```python
from build123d import *

# Parameters (mm, degrees)
SKETCH_1_R               = 275
SKETCH_1_R_2             = 255
EXTRUDE_1_DEPTH          = 10
EXTRUDE_2_DEPTH          = 10
SKETCH_8_R               = 2.65
SKETCH_8_R_2             = 2.15
CUT_EXTRUDE_1_DEPTH      = 21
SKETCH_9_OUTSIDE_W       = 707.614
SKETCH_9_OUTSIDE_H       = 707.614
CUT_EXTRUDE_2_DEPTH      = 21
SKETCH_10_W              = 190.987823936
SKETCH_10_H              = 12
CUT_EXTRUDE_3_DEPTH      = 519.420037555
CUT_EXTRUDE_3_DEPTH_BACK = 245.939436413
FILLET_1_R               = 3
FILLET_2_R               = 10
FILLET_3_R               = 5
SKETCH_11_W              = 751.740061758
SKETCH_11_H              = 25.075171634
CUT_EXTRUDE_4_DEPTH      = 519.420037555
CUT_EXTRUDE_4_DEPTH_BACK = 245.939436413


with BuildPart() as part:
    # 草图1 → 凸台-拉伸1 (new body)
    with BuildSketch(Plane(origin=(0, 0, 0), x_dir=(1, 0, 0), z_dir=(0, 1, 0))):
        Circle(SKETCH_1_R)
        Circle(SKETCH_1_R_2, mode=Mode.SUBTRACT)
    extrude(amount=EXTRUDE_1_DEPTH)

    # 草图11 → 切除-拉伸4 (cut, two sides)
    with BuildSketch(Plane(origin=(76.33674701, 0, -113.448714652), x_dir=(0.829665535, 0, 0.558260781), z_dir=(-0.558260781, 0, 0.829665535))) as cut_extrude_4_sk:
        with Locations((71.776229786, 3.462414183)):
            Rectangle(SKETCH_11_W, SKETCH_11_H)
    extrude(amount=CUT_EXTRUDE_4_DEPTH, mode=Mode.SUBTRACT)
    extrude(cut_extrude_4_sk.sketch, amount=-CUT_EXTRUDE_4_DEPTH_BACK, mode=Mode.SUBTRACT)


with BuildPart() as body_2:
    # 草图2 → 凸台-拉伸2 (new body)
    with BuildSketch(Plane(origin=(0, 10, 0), x_dir=(1, 0, 0), z_dir=(0, 1, 0))):
        with BuildLine():
            Line((-110.525139894, 257.262887824), (-25.423255477, 200))
            Line((-25.423255477, 200), (0, 200))
            Line((0, 200), (25.423255477, 200))
            Line((25.423255477, 200), (110.525139894, 257.262887824))
            ThreePointArc((110.525139894, 257.262887824), (197.989898732, 197.989898732), (257.262887824, 110.525139894))
            Line((257.262887824, 110.525139894), (200, 25.423255477))
            Line((200, 25.423255477), (200, 0))
            Line((200, 0), (200, -25.423255477))
            Line((200, -25.423255477), (257.262887824, -110.525139894))
            ThreePointArc((257.262887824, -110.525139894), (197.989898732, -197.989898732), (110.525139894, -257.262887824))
            Line((110.525139894, -257.262887824), (25.423255477, -200))
            Line((25.423255477, -200), (0, -200))
            Line((0, -200), (-25.423255477, -200))
            Line((-25.423255477, -200), (-110.525139894, -257.262887824))
            ThreePointArc((-110.525139894, -257.262887824), (-197.989898732, -197.989898732), (-257.262887824, -110.525139894))
            Line((-257.262887824, -110.525139894), (-200, -25.423255477))
            Line((-200, -25.423255477), (-200, 25.423255477))
            Line((-200, 25.423255477), (-257.262887824, 110.525139894))
            ThreePointArc((-257.262887824, 110.525139894), (-197.989898732, 197.989898732), (-110.525139894, 257.262887824))
        make_face()
        with BuildLine():
            Line((0, 185), (30, 185))
            Line((30, 185), (111.993839361, 240.171563565))
            ThreePointArc((111.993839361, 240.171563565), (187.383297014, 187.383297014), (240.171563565, 111.993839361))
            Line((240.171563565, 111.993839361), (185, 30))
            Line((185, 30), (185, 0))
            Line((185, 0), (185, -30))
            Line((185, -30), (240.171563565, -111.993839361))
            ThreePointArc((240.171563565, -111.993839361), (187.383297014, -187.383297014), (111.993839361, -240.171563565))
            Line((111.993839361, -240.171563565), (30, -185))
            Line((30, -185), (0, -185))
            Line((0, -185), (-30, -185))
            Line((-30, -185), (-111.993839361, -240.171563565))
            ThreePointArc((-111.993839361, -240.171563565), (-187.383297014, -187.383297014), (-240.171563565, -111.993839361))
            Line((-240.171563565, -111.993839361), (-185, -30))
            Line((-185, -30), (-185, 30))
            Line((-185, 30), (-240.171563565, 111.993839361))
            ThreePointArc((-240.171563565, 111.993839361), (-187.383297014, 187.383297014), (-111.993839361, 240.171563565))
            Line((-111.993839361, 240.171563565), (-30, 185))
            Line((-30, 185), (0, 185))
        make_face(mode=Mode.SUBTRACT)
    extrude(amount=EXTRUDE_2_DEPTH)

    # 草图8 → 切除-拉伸1 (cut, through all)
    with BuildSketch(Plane(origin=(0, 20, 0), x_dir=(1, 0, 0), z_dir=(0, 1, 0))):
        with Locations((-10, 192.5)):
            Circle(SKETCH_8_R)
        with Locations((10, 192.5)):
            Circle(SKETCH_8_R)
        with Locations((-10, -192.5)):
            Circle(SKETCH_8_R)
        with Locations((10, -192.5)):
            Circle(SKETCH_8_R)
        with Locations((192.5, 10)):
            Circle(SKETCH_8_R)
        with Locations((192.5, -10)):
            Circle(SKETCH_8_R)
        with Locations((-192.5, 10)):
            Circle(SKETCH_8_R)
        with Locations((-192.5, -10)):
            Circle(SKETCH_8_R)
        with Locations((-110.525139894, 248.223100485)):
            Circle(SKETCH_8_R_2)
        with Locations((-27.711627738, 192.5)):
            Circle(SKETCH_8_R_2)
        with Locations((-44.304938442, 203.665215623)):
            Circle(SKETCH_8_R_2)
        with Locations((-56.749921469, 212.03912734)):
            Circle(SKETCH_8_R_2)
        with Locations((-69.194904497, 220.413039057)):
            Circle(SKETCH_8_R_2)
        with Locations((-81.639887524, 228.786950774)):
            Circle(SKETCH_8_R_2)
        with Locations((-146.077022117, 230.028561882)):
            Circle(SKETCH_8_R_2)
        with Locations((-164.415519771, 217.299729706)):
            Circle(SKETCH_8_R_2)
        with Locations((-183.638937552, 201.316607082)):
            Circle(SKETCH_8_R_2)
        with Locations((-201.316607082, 183.638937552)):
            Circle(SKETCH_8_R_2)
        with Locations((-217.299729706, 164.415519771)):
            Circle(SKETCH_8_R_2)
        with Locations((-230.028561882, 146.077022117)):
            Circle(SKETCH_8_R_2)
        with Locations((-128.811575358, 240.123330241)):
            Circle(SKETCH_8_R)
        with Locations((-240.123330241, 128.811575358)):
            Circle(SKETCH_8_R)
        with Locations((-228.786950774, 81.639887524)):
            Circle(SKETCH_8_R_2)
        with Locations((-220.413039057, 69.194904497)):
            Circle(SKETCH_8_R_2)
        with Locations((-212.03912734, 56.749921469)):
            Circle(SKETCH_8_R_2)
        with Locations((-203.665215623, 44.304938442)):
            Circle(SKETCH_8_R_2)
        with Locations((-192.5, 27.711627738)):
            Circle(SKETCH_8_R_2)
        with Locations((-248.223100485, 110.525139894)):
            Circle(SKETCH_8_R_2)
        with Locations((192.5, 27.711627738)):
            Circle(SKETCH_8_R_2)
        with Locations((248.223100485, 110.525139894)):
            Circle(SKETCH_8_R_2)
        with Locations((203.665215623, 44.304938442)):
            Circle(SKETCH_8_R_2)
        with Locations((212.03912734, 56.749921469)):
            Circle(SKETCH_8_R_2)
        with Locations((220.413039057, 69.194904497)):
            Circle(SKETCH_8_R_2)
        with Locations((228.786950774, 81.639887524)):
            Circle(SKETCH_8_R_2)
        with Locations((240.123330241, 128.811575358)):
            Circle(SKETCH_8_R)
        with Locations((230.028561882, 146.077022117)):
            Circle(SKETCH_8_R_2)
        with Locations((128.811575358, 240.123330241)):
            Circle(SKETCH_8_R)
        with Locations((201.316607082, 183.638937552)):
            Circle(SKETCH_8_R_2)
        with Locations((183.638937552, 201.316607082)):
            Circle(SKETCH_8_R_2)
        with Locations((164.415519771, 217.299729706)):
            Circle(SKETCH_8_R_2)
        with Locations((146.077022117, 230.028561882)):
            Circle(SKETCH_8_R_2)
        with Locations((81.639887524, 228.786950774)):
            Circle(SKETCH_8_R_2)
        with Locations((69.194904497, 220.413039057)):
            Circle(SKETCH_8_R_2)
        with Locations((56.749921469, 212.03912734)):
            Circle(SKETCH_8_R_2)
        with Locations((44.304938442, 203.665215623)):
            Circle(SKETCH_8_R_2)
        with Locations((110.525139894, 248.223100485)):
            Circle(SKETCH_8_R_2)
        with Locations((27.711627738, 192.5)):
            Circle(SKETCH_8_R_2)
        with Locations((217.299729706, 164.415519771)):
            Circle(SKETCH_8_R_2)
    extrude(amount=-CUT_EXTRUDE_1_DEPTH, mode=Mode.SUBTRACT)

    # 草图9 outside → 切除-拉伸2 (cut, through all)
    with BuildSketch(Plane(origin=(0, 20, 0), x_dir=(1, 0, 0), z_dir=(0, 1, 0))):
        Rectangle(SKETCH_9_OUTSIDE_W, SKETCH_9_OUTSIDE_H)
        with BuildLine():
            Line((-157.049761777, 231.808913387), (-146.237600169, 220.996751779))
            ThreePointArc((-146.237600169, 220.996751779), (-129.47118383, 231.218971016), (-111.993839361, 240.171563565))
            Line((-111.993839361, 240.171563565), (-64.194904497, 208.008879225))
            Line((-64.194904497, 208.008879225), (-64.194904497, 226.088453902))
            Line((-64.194904497, 226.088453902), (-110.525139894, 257.262887824))
            ThreePointArc((-110.525139894, 257.262887824), (-134.391436501, 245.639861983), (-157.049761777, 231.808913387))
        make_face(mode=Mode.SUBTRACT)
    extrude(amount=-CUT_EXTRUDE_2_DEPTH, mode=Mode.SUBTRACT)

    # 草图10 → 切除-拉伸3 (cut, two sides)
    with BuildSketch(Plane(origin=(76.33674701, 0, -113.448714652), x_dir=(0.829665535, 0, 0.558260781), z_dir=(-0.558260781, 0, 0.829665535))) as cut_extrude_3_sk:
        with Locations((-226.995793353, 10)):
            Rectangle(SKETCH_10_W, SKETCH_10_H)
    extrude(amount=CUT_EXTRUDE_3_DEPTH, mode=Mode.SUBTRACT)
    extrude(cut_extrude_3_sk.sketch, amount=-CUT_EXTRUDE_3_DEPTH_BACK, mode=Mode.SUBTRACT)

    # 圆角1
    fillet_1_edges = [body_2.edges().sort_by_distance(p)[0] for p in [
        (-64.194904497, 18, -208.008879225),
    ]]
    fillet(fillet_1_edges, radius=FILLET_1_R)

    # 圆角2
    fillet_2_edges = [body_2.edges().sort_by_distance(p)[0] for p in [
        (-110.525139894, 18, -257.262887824),
        (-111.993839361, 18, -240.171563565),
    ]]
    fillet(fillet_2_edges, radius=FILLET_2_R)

    # 圆角3
    fillet_3_edges = [body_2.edges().sort_by_distance(p)[0] for p in [
        (-146.237600169, 18, -220.996751779),
        (-64.194904497, 18, -226.088453902),
        (-157.049761777, 18, -231.808913387),
    ]]
    fillet(fillet_3_edges, radius=FILLET_3_R)


solid = body_2.part
```
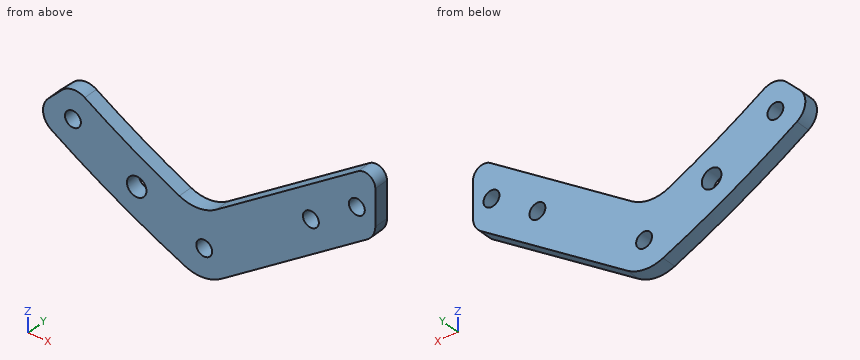
Work out the finished part from the listing and answer in its coordinate system (mm). Coordinates: 2 decimals unless noted, no trailing zeros. Write each loop counter-clockwise with the first axis right and the second up, starting at its lowest first coordinate (ties: lowest second). Pieces come first, ordered by that corner, then holes.
Q1. A cutting plane is placed at B-B, the plane z = -219.5. Give the vertices of the cut face in (x, y).
Q2. Each of these flat-tipped pins is pushed along its axis until it touches: pin 1 Ø2 at (x, y) = (-74.5, 18) entering from -Z; pin 2 Ø1.5 at (y, z) = (18, -249.5) entering from -X; pin 3 Ø1 at (x, y) = (-110, 17.5) entering from +Z. Where does it stop, or does it pass through?
Q3. A cutting plane is placed at C-C, the plane y = 17.7. Give the vertices of the cut face in (x, z), then the cut area to 3 significant figures.
Q4. A cutting plane is placed at D-D, the plane x = -93. Give the vertices of the cut face in (y, z), then the cut area to 3 significant figures.
Q5. A cutting plane is placed at A-A, the plane x = -110. Give the vertices of the cut face in (y, z), then the cut area to 3 significant figures.
Q6. Find the intervals of material crossed by line 1 (X direction, y = 17.9, z = -228.5); line 2 (X direction, y = 17.75, z = -227); line 3 (X direction, y = 18.5, z = -235), in increasing order.
Findings below:
1. outline: (-81.27, 16) - (-71.14, 16) - (-71.14, 20) - (-81.27, 20) - close; (-67.25, 16) - (-64.19, 16) - (-64.19, 20) - (-67.25, 20) - close
2. pin 1: stops at z = -233.7
2. pin 2: stops at x = -128.54
2. pin 3: stops at z = -238.11
3. outline: (-152.72, -227.48) arc R5 ccw to (-151.9, -235.22) arc R280 ccw to (-115.66, -254.99) arc R10 ccw to (-105.95, -254.18) - (-66.4, -227.57) arc R5 ccw to (-64.19, -223.43) - (-64.19, -213.64) arc R3 ccw to (-68.87, -211.15) - (-107.25, -236.98) arc R10 cw to (-117.25, -237.65) arc R265 cw to (-142.87, -223.19) arc R5 ccw to (-149.1, -223.86) - close; hole circle Ø4.3 at (-146.08, -230.03); hole circle Ø5.3 at (-128.81, -240.12); hole circle Ø4.3 at (-110.53, -248.22); hole circle Ø4.3 at (-81.64, -228.79); hole circle Ø4.3 at (-69.19, -220.41)
3. area: 1,440 mm2
4. outline: (16, -245.47) - (20, -245.47) - (20, -227.39) - (16, -227.39) - close
4. area: 72.3 mm2
5. outline: (16, -255.77) - (20, -255.77) - (20, -250.31) - (16, -250.31) - close; (16, -246.14) - (20, -246.14) - (20, -238.27) - (16, -238.27) - close
5. area: 53.3 mm2
6. line 1: x = -153.51 to -147.59, -144.57 to -134.21, -94.65 to -83.77, -79.51 to -67.78
6. line 2: x = -152.24 to -136.73, -92.42 to -82.84, -80.44 to -65.7
6. line 3: x = -152.21 to -122.47, -104.31 to -77.44
